Autodesk Inventor part; units mm, degrees
ref_plane "YZ Plane" through (0, 0, 0) normal (1, 0, 0) x (0, 1, 0)
ref_plane "XZ Plane" through (0, 0, 0) normal (0, 1, 0) x (-1, 0, 0)
ref_plane "XY Plane" through (0, 0, 0) normal (0, 0, 1) x (1, 0, 0)
sketch "Sketch1" plane through (0, 0, 0) normal (0, 0, 1) x (1, 0, 0)
  line L0 (0, 2.65) -> (0, -2.65)
  line L1 (-1.85, 0) -> (1.85, 0)
  line L2 (1.85, 1.8974) -> (1.85, -1.8974)
  arc A0 (1.85, 1.8974) -> (-1.85, 1.8974) centre (0, 0) ccw
  line L3 (-1.85, 1.8974) -> (-1.85, -1.8974)
  arc A1 (-1.85, -1.8974) -> (1.85, -1.8974) centre (0, 0) ccw
  line L4 (0, 0) -> (45, 0) construction
  line L5 (0, -6) -> (45, -6)
  line L6 (45, 6) -> (0, 6)
  arc A2 (0, 6) -> (0, -6) centre (0, 0) ccw
  arc A3 (45, -6) -> (45, 6) centre (45, 0) ccw
  point P0 (22.5, 0)
  dimension "d0" = 2.65
  dimension "d1" = 3.7
  dimension "d2" = 6
  dimension "d3" = 45
extrude "Plate1" add sketch "Sketch1" along normal blind 3
equation "\"d4\" = Thickness"
equation "\"BendRadius\" = Thickness"
equation "\"BendReliefWidth\" = Thickness"
equation "\"BendReliefDepth\" = 0.5 * Thickness"
equation "\"CornerReliefSize\" = 4 * Thickness"
equation "\"MinimumRemnant\" = 2 * Thickness"
equation "\"TransitionRadius\" = BendRadius"
equation "\"JacobiRadiusSize\" = BendRadius"
equation "\"GapSize\" = Thickness"
properties part number "Shooting Arm V2"
Design review of the part built by this model. Coordinates are the model's own, in mm. A direction names the side the tool comes from. Give positions to 0.01 mm unless a question says otherwise; leave off trailing zeros. Write each loop counter-clockwise with the first axis right and the second up, starting at its lowest first coordinate (ties: lowest second). Pieces come first, ordered by that corner, then holes. Notation, with made-up numbers: (-29, 15.5) - (0, 15.5) arc R16 ccw to (0, 46.5) - close; hole circle Ø7 at (52, 34). An arc over 180 degrees is marked (long way). Return JSON: item names as keys, results as strings. Group by question number.
(1) Insertion check: pin 1 (0.9 mm diameter, centred on y = -1, z = 1.5, fed in from +X). The pin has a flat end and moves straight along its axis. Give the tip position at first contact, or say it passes through.
(2) We need section B-B, the plane y = 0. Give the boundary of the cut face in (x, z), then the cut area to 3 significant figures.
(3) Mouldability with a two-part tool opening along Y and no side actions: class faces 3 (the flat face through (22, 0, 3)), 4 (the flat face through (1.85, 0, 1)), 5 (the cylindrical face through (-6, 0, 1)) as +Y half, -Y half, draft (parallel to the pull), parting line (faces both ways), or undercut.
(4) We need section C-C, the plane y = 4.5. Give the boundary of the cut face in (x, z), then the cut area to 3 significant figures.
(5) We need section A-A, the plane z = 0.6. Give the boundary of the cut face in (x, y).
(6) Machinability: for faces 1 (the cylindrical face through (0.03, -2.65, 1.48)), 2 (the flat face through (23, 6, 1)), which of the approach directions +Z, -Z, +X, -X, +Y, -Y give a long, thin tool a straight path to every point of the face, cutting with its end or side? Answer none if there is none.
(7) To check wall thickness, follow probe 1 along X at (y, z) = (0, 2.8); probe 2 along X at (y, z) = (-2, 0.95); probe 3 along X at (y, z) = (5.25, 1.1). State the ranges of each line that lie inside material, in increasing order.
Reported:
{
 "1": {"pin 1": "stops at x = 50.97"},
 "2": {"outline": "(-6, 0) - (-1.85, 0) - (-1.85, 3) - (-6, 3) - close; (1.85, 0) - (51, 0) - (51, 3) - (1.85, 3) - close", "area": "160 mm2"},
 "3": {"face 3": "draft", "face 4": "undercut", "face 5": "parting line"},
 "4": {"outline": "(-3.97, 0) - (48.97, 0) - (48.97, 3) - (-3.97, 3) - close", "area": "159 mm2"},
 "5": {"outline": "(0, -6) - (45, -6) arc R6 ccw to (45, 6) - (0, 6) arc R6 ccw to start; hole (-1.85, -1.9) arc R2.65 ccw to (1.85, -1.9) - (1.85, 1.9) arc R2.65 ccw to (-1.85, 1.9) - close"},
 "6": {"face 1": "+Z, -Z", "face 2": "+Z, -Z, +X, -X, +Y"},
 "7": {"probe 1": "x = -6 to -1.85, 1.85 to 51", "probe 2": "x = -5.66 to -1.74, 1.74 to 50.66", "probe 3": "x = -2.9 to 47.9"}
}
